Build history of the part. All positions in model axes, mm. A direction names the side the tool comes from. Round coordinates to 2 decimals unless told otherwise and drop trailing zeros. Order: outer loops, then holes, each group sorted by start corner. A loop starts at its lowest first (then second) coordinate and runs counter-clockwise, first axis right, second up. Notation, with made-up numbers: (51.25, -24.75) -> (102.25, -24.75) arc R25 ccw to (102.25, -1.75) -> close; hole circle Ø6 at (9, 17.5). An arc over 180 degrees is marked (long way). Answer as a JSON object with one key per item and string values.
from build123d import *

# Parameters (mm, degrees)
SKETCH3_R          = 3.175
CUT_EXTRUDE1_DEPTH = 15.893870686


with BuildPart() as part:
    # Sketch2 → Barbfitting(Mcmaster) (revolve)
    with BuildSketch(Plane(origin=(0, 0, 0), x_dir=(0, 0, -1), z_dir=(1, 0, 0))):
        Polygon((8.7391875, 0), (-6.154683186, 0), (-6.154683186, 4.205934994), (-6.005566814, 4.223690006), (-1.554901936, 4.753622494), (-1.554901936, 4.205934994), (-1.405785564, 4.223690006), (3.044879314, 4.753622494), (3.044879314, 4.205934994), (3.193995686, 4.223690006), (7.707996691, 4.76116381), (8.7391875, 4.7625), align=None)
    revolve(axis=Axis((0, 0, -8.7391875), (0, 0, 1)))

    # Sketch3 → Cut-Extrude1 (cut, through all)
    with BuildSketch(Plane.XY.offset(6.154683186)):
        Circle(SKETCH3_R)
    extrude(amount=-CUT_EXTRUDE1_DEPTH, mode=Mode.SUBTRACT)


solid = part.part
1) Cut at B-B, the plane z = -3.75. Give the cut face in (x, y) (3 decimals).
Checked values:
{"outline": "circle Ø8.58 at (0, 0); hole circle Ø6.35 at (0, 0)"}
2) Which spindle directions (+Z, -Z, +X, -X, +Y, -Y) get a long thin tool onto all of the face, cutting with end or side? Do faces 1 (the face through (-3, 2, 6.155)), 2 (the face through (4, 2, -3.045)). Say none if no direction does.
Checked values:
{"face 1": "+Z, +X, -X, +Y, -Y", "face 2": "none"}
3) Pull direction X, two halves, no side cores. Call faces 3 (the face through (-0.69, -3.1, -1.19)), 4 (the face through (4.65, -1.03, -8.23)), 5 (the face through (4, 2, 1.555)): pulls with the +X half, pulls with the -X half, needs draft (parallel to the pull), parting line crosses it, or undercut.
Checked values:
{"face 3": "undercut", "face 4": "parting line crosses it", "face 5": "needs draft"}
4) Cut at A-A, the plane z = 1.75. Give the cut face in (x, y) (3 decimals).
Checked values:
{"outline": "circle Ø9.461 at (0, 0); hole circle Ø6.35 at (0, 0)"}
5) Flat gauge pins, fed straight in: pin 1 Ø1.5 at (y, z) = (1, -5) entering from -X; pin 2 Ø2 at (x, z) = (2.5, 3) entering from +Y; pin 3 Ø3 at (y, z) = (-1, -3.5) entering from +X; pin 4 Ø3 at (x, y) = (0, 0) entering from -Z. Where does each tip first touch, or does it go through?
Checked values:
{"pin 1": "stops at x = -4.48", "pin 2": "stops at y = 4.35", "pin 3": "stops at x = 4.75", "pin 4": "passes through"}
6) Probe L1, parallel to Y at x = 1.75, z = 4; L2, parallel to X at y = 2.25, z = 1.25; L3, parallel to Y at x = 0, z = 1.75 (3 decimals). List the from-to ranges inside material, lowest first. Write a range as from..to.
Checked values:
{"L1": "y = -4.11..-2.65, 2.65..4.11", "L2": "x = -3.6..-2.24, 2.24..3.6", "L3": "y = -4.73..-3.175, 3.175..4.73"}
